from build123d import *

# Parameters (mm, degrees)
SKETCH_1_R          = 13
EXTRUDE_1_DEPTH     = 17.5
SKETCH_2_R          = 10
CUT_EXTRUDE_1_DEPTH = 17.5
CHAMFER_1_SIZE      = 0.5


with BuildPart() as part:
    # 草图1 → 凸台-拉伸1 (new body)
    with BuildSketch(Plane.XY):
        Circle(SKETCH_1_R)
    extrude(amount=EXTRUDE_1_DEPTH)

    # 草图2 → 切除-拉伸1 (cut)
    with BuildSketch(Plane.XY.offset(17.5)):
        Circle(SKETCH_2_R)
    extrude(amount=-CUT_EXTRUDE_1_DEPTH, mode=Mode.SUBTRACT)

    # 倒角1
    chamfer_1_edges = [part.edges().sort_by_distance(p)[0] for p in [
        (-13, 0, 0),
        (-13, 0, 17.5),
    ]]
    chamfer(chamfer_1_edges, length=CHAMFER_1_SIZE)


solid = part.part
Verification items for the finished model (mm, model axes). Round coordinates to 2 decimals unless told otherwise and drop trailing zeros. Loops run counter-clockwise (first coordinate to the right, second up) from the corner with the lowest first, then second, coordinate; pieces in that order, holes last. Notation, with made-up numbers: M -26,64.5 L 22,64.5 A24 ccw 22,84.5 Z; hole C 68.25,64.5 d9. An arc over 180 degrees is marked long. Write each question's results on one line, items separated by ' | '.
1) Mould release check, pull along X, two halves, no side actions. Record for faces 1 (the cylindrical face through (-2.17, -9.76, 8.87)), 2 (the flat face through (-0.1, 10.2, 17.5)), 3 (the cylindrical face through (-10.316, -7.91, 8.634)): released by +X, released by -X, zero draft, split by the parting line, or undercut.
Checks:
face 1: undercut | face 2: zero draft | face 3: split by the parting line
2) Scan lines: L1, parallel to Y at x = 0, z = 10.25; L2, parallel to Y at x = 9, z = 6.25; L3, parallel to X at y = -6.5, z = 1. Record each from-to range of solid material in increasing order. Write a range as from..to.
Checks:
L1: y = -13..-10, 10..13 | L2: y = -9.38..-4.36, 4.36..9.38 | L3: x = -11.26..-7.6, 7.6..11.26
3) Section check C-C on z = 15.25. Record the boundary of the cut face in (x, y).
Checks:
outline: C 0,0 d26; hole C 0,0 d20
4) Section check A-A on x = 0. Record the boundary of the cut face in (y, z).
Checks:
outline: M -13,0.5 L -12.5,0 L -10,0 L -10,17.5 L -12.5,17.5 L -13,17 Z; M 10,0 L 12.5,0 L 13,0.5 L 13,17 L 12.5,17.5 L 10,17.5 Z
5) Gauge pin test, flat ends, axial feed: P1, Ø6, axis at x = 6, z = 8, coming from the +Y side; P2, Ø4, axis at x = -8.5, z = 13.5, coming from the +Y side; P3, Ø10, axis at x = -7.5, z = 5, coming from the +Y side. Record the tip position at first contact, or that the pin passes through.
Checks:
P1: stops at y = 12.65 | P2: stops at y = 11.26 | P3: stops at y = 12.76
